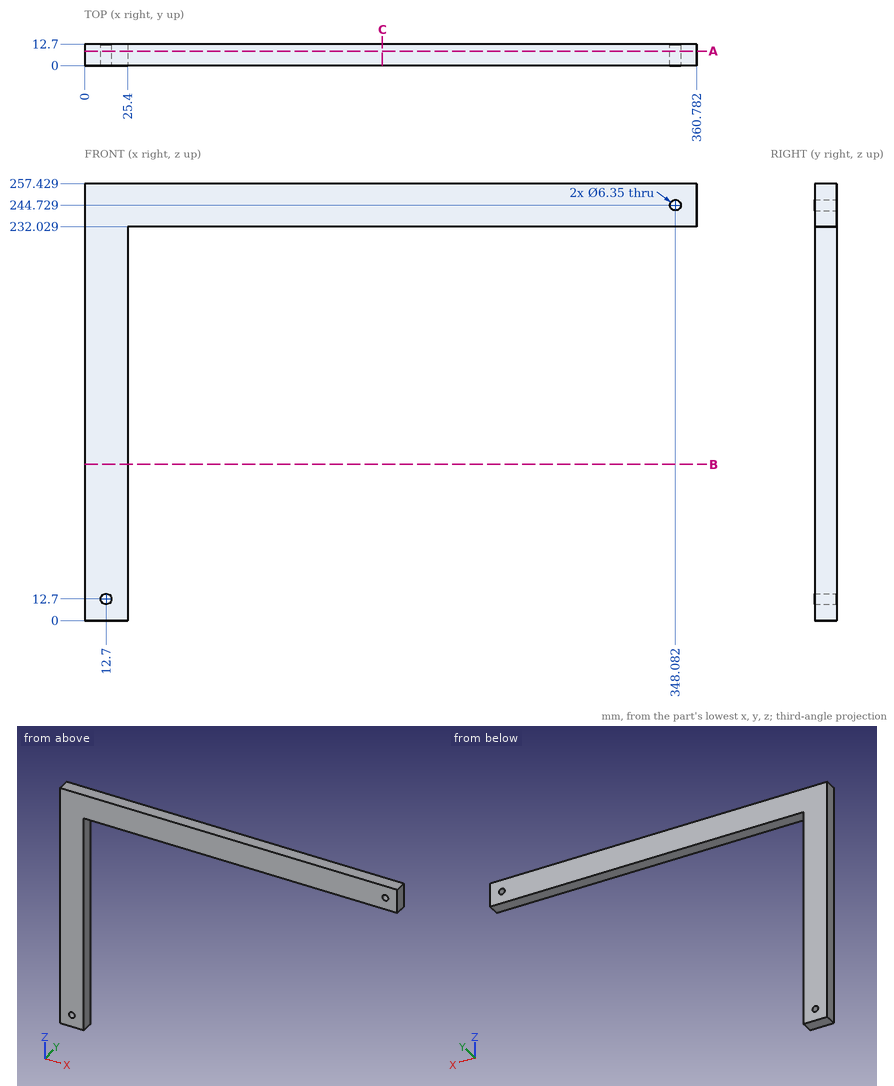
Study the drawing (mm; zero at the part's minimum x, y, z) and answer. Coordinates: 2 decimals unless noted, no trailing zeros. Loops run counter-clockwise (first coordinate to the right, second up) from the corner with the lowest first, then second, coordinate; pieces in that order, holes last. Notation, with made-up numbers: (47.5, 81.5) -> (79.5, 81.5) arc R8 ccw to (79.5, 95.5) -> close; hole circle Ø3 at (23.5, 26.5). An arc over 180 degrees is marked (long way). Answer in a Markdown table with one row per item. Add a question column.
1. The part is cut by section C-C, the plane x = 175.5. Write down the section's boundary in (y, z), then the cut area to 3 significant figures.
2. The part is cut by section A-A, the plane y = 8.5. Count the separate pieces of the cut face and the enclosed holes in it, then the cut area to 3 significant figures.
3. The part is cut by section B-B, the plane z = 92. Write down the section's boundary in (x, y).
4. Consider line 1 (Z direction, x = 12.7, y = 7.5) (1 decimal); line 2 (Z direction, x = 195, y = 4.75); line 3 (X direction, y = 11.25, z = 177.5). Determine where each line is inside the solid, lowest interval first. Write a range as [from, to].
5. Flat-ended cylindrical pins translate along their axes: P1, Ø10, axis at x = 348.08, z = 244.73, coming from the +Y side; P2, Ø3, axis at x = 191, y = 1.5, coming from the -Z side. Find the tip coordinate at first contact, or state that the pin passes through.
Answer below:
| question | item | result |
|---|---|---|
| 1 | outline | (0, 232.03) -> (12.7, 232.03) -> (12.7, 257.43) -> (0, 257.43) -> close |
| 1 | area | 323 mm2 |
| 2 | separate pieces | 1 |
| 2 | enclosed holes | 2 |
| 2 | area | 15,000 mm2 |
| 3 | outline | (0, 0) -> (25.4, 0) -> (25.4, 12.7) -> (0, 12.7) -> close |
| 4 | line 1 | [0, 9.5], [15.9, 257.4] |
| 4 | line 2 | [232.03, 257.43] |
| 4 | line 3 | [0, 25.4] |
| 5 | P1 | y = 12.7 |
| 5 | P2 | z = 232.03 |
